Geometry check sheet. Reference: the model listing, model coordinates, mm. Face numbers are marked on the shaded views. A direction names the side the tool comes from. Round coordinates to 2 decimals unless told otherwise and drop trailing zeros. Order: outer loops, then holes, each group sorted by start corner. A loop starts at its lowest first (then second) coordinate and runs counter-clockwise, first axis right, second up. Notation, with made-up numbers: (58.25, 23) - (106.25, 23) arc R22 ccw to (106.25, 35) - close; hole circle Ø1 at (54.5, -20.5). An arc over 180 degrees is marked (long way). Return JSON: item names as keys, results as strings. Group by question number.
Q1. Sectioned sample at A-A, the plane z = 10. Record the cut outline in (x, y).
Q2. Gauge pin test, flat ends, axial feed: pin 1 Ø4.5 at (x, z) = (-20, 10) entering from +Y; pin 2 Ø11 at (x, y) = (-11.5, 30) entering from -Z; pin 3 Ø4 at (x, z) = (13.5, 22) entering from +Y. Record the tip position at first contact, or that the pin passes through.
Q3. Sectioned sample at B-B, the plane x = 20. Record the cut outline in (y, z), then the cut area to 3 significant figures.
Q4. Material ranges on line 1 along X through (y, z) = (2.65, 10); line 2 along Z through (x, y) = (20, 2.8); line 3 along Y through (x, z) = (-21, 24.5), recorded low to high.
Q5. Tool access check on the marked faces 1 and 2. Record the directions out of +Z, -Z, +X, -X, +Y, -Y that give a thin tool (end or side, any length) a straight path to the whole face; none if there is none.
Q6. Sectioned sample at C-C, the plane x = -27. Record the cut outline in (y, z), then the cut area to 3 significant figures.
Q7. Sectioned sample at D-D, the plane z = 17. Record the cut outline in (x, y), then the cut area to 3 significant figures.
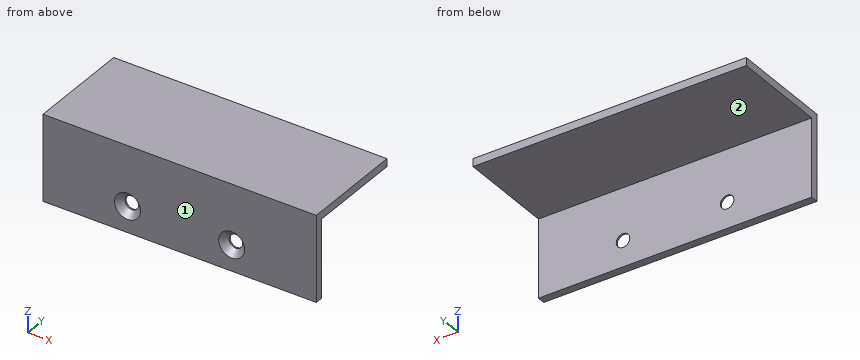
Autodesk Inventor part; units mm, degrees
ref_plane "YZ Plane" through (0, 0, 0) normal (1, 0, 0) x (0, 1, 0)
ref_plane "XZ Plane" through (0, 0, 0) normal (0, 1, 0) x (-1, 0, 0)
ref_plane "XY Plane" through (0, 0, 0) normal (0, 0, 1) x (1, 0, 0)
sketch "Skizze1" plane through (0, 0, 0) normal (1, 0, 0) x (0, 1, 0)
  line L0 (0, 0) -> (3, 0)
  line L1 (3, 0) -> (3, 30)
  line L2 (3, 30) -> (0, 30)
  line L3 (0, 30) -> (0, 0)
  line L4 (0, 30) -> (40, 30)
  line L5 (40, 30) -> (40, 33)
  line L6 (40, 33) -> (0, 33)
  line L7 (0, 33) -> (0, 30)
  dimension "d1" = 3
  dimension "d2" = 30
  dimension "d3" = 40
  dimension "d4" = 3
extrude "Extrusion1" add sketch "Skizze1" along normal mid plane 105
sketch "Skizze2" plane through (-52.5, 0, 0) normal (0, -1, 0) x (1, 0, 0)
  line L0 (10.5897, 10) -> (79.1743, 10) construction
  line L1 (0, 0) -> (105, 0) construction
  line L2 (52.5, 0) -> (52.5, 22.0905) construction
  point P0 (32.5, 10)
  point P1 (72.5, 10)
  dimension "d7" = 10
  dimension "d8" = 20
hole "Bohrung1" at (-20, 0, 10) at (20, 0, 10) direction (0, 1, 0) diameter 5.2 end through all countersink diameter 10 countersink angle 90
equation "\"d5\" = Magazin_Breite"
equation "\"Magazin_Breite\" = 105"
properties part number "TS_Magazin_Begrenzung_int"
Reply:
{
 "1": {"outline": "(-52.5, 0) - (-25, 0) - (-22.6, 2.4) - (-22.6, 3) - (-52.5, 3) - close; (-17.4, 2.4) - (-15, 0) - (15, 0) - (17.4, 2.4) - (17.4, 3) - (-17.4, 3) - close; (22.6, 2.4) - (25, 0) - (52.5, 0) - (52.5, 3) - (22.6, 3) - close"},
 "2": {"pin 1": "through", "pin 2": "z = 30", "pin 3": "y = 3"},
 "3": {"outline": "(0, 0) - (3, 0) - (3, 7.4) - (2.4, 7.4) - (0, 5) - close; (0, 15) - (2.4, 12.6) - (3, 12.6) - (3, 30) - (40, 30) - (40, 33) - (0, 33) - close", "area": "189 mm^2"},
 "4": {"line 1": "-52.5 to -22.6, -17.4 to 17.4, 22.6 to 52.5", "line 2": "0 to 7.4, 12.6 to 33", "line 3": "0 to 3"},
 "5": {"face 1": "+Z, -Z, +X, -X, -Y", "face 2": "-Z, +X, -X, +Y"},
 "6": {"outline": "(0, 0) - (3, 0) - (3, 30) - (40, 30) - (40, 33) - (0, 33) - close", "area": "210 mm^2"},
 "7": {"outline": "(-52.5, 0) - (52.5, 0) - (52.5, 3) - (-52.5, 3) - close", "area": "315 mm^2"}
}
